Geometry: final body of the model. Coordinates: model frame, mm. A direction names the side the tool comes from. Give positions to 0.01 mm unless a question says otherwise; leave off trailing zeros. Write each loop counter-clockwise with the first axis right and the second up, starting at its lowest first coordinate (ties: lowest second). Pieces come first, ordered by that corner, then holes.
```python
from build123d import *
from build123d.topology import SkipClean

# Parameters (mm, degrees)
BOSS_EXTRUDE1_DEPTH  = 19.05
CUT_EXTRUDE1_DEPTH   = 12.7
MIRROR2_COPY_1_DEPTH = 12.7
SKETCH6_W            = 6.35
SKETCH6_H            = 32.8168
SKETCH6_W_2          = 32.8168
SKETCH6_H_2          = 6.35
CUT_EXTRUDE2_DEPTH   = 12.7
SKETCH7_R            = 0.675
BOSS_EXTRUDE2_DEPTH  = 12.7
FILLET2_DEPTH        = 20
CUT_EXTRUDE3_DEPTH   = 12.7


with BuildPart() as part:
    # Sketch5 → Boss-Extrude1 (new body)
    with BuildSketch(Plane.XY):
        with BuildLine():
            Line((-15.875, 15.875), (-15.875, -15.875))
            Line((-15.875, -15.875), (15.875, -15.875))
            ThreePointArc((15.875, -15.875), (26.071916674, -9.061638106), (38.1, -6.669103576))
            Line((38.1, -6.669103576), (38.1, 6.669103576))
            ThreePointArc((38.1, 6.669103576), (15.875, 15.875), (6.669103576, 38.1))
            Line((6.669103576, 38.1), (-6.669103576, 38.1))
            ThreePointArc((-6.669103576, 38.1), (-9.061638106, 26.071916674), (-15.875, 15.875))
        make_face()
    extrude(amount=BOSS_EXTRUDE1_DEPTH)

    # Sketch4 → Cut-Extrude1 (cut)
    with BuildSketch(Plane.XY):
        with BuildLine():
            Line((4.190365, -12.7), (10.11729625, -12.7))
            Line((10.11729625, -12.7), (12.7, -12.7))
            Line((12.7, -12.7), (12.7, -10.11729625))
            Line((12.7, -10.11729625), (12.7, -4.190365))
            Line((12.7, -4.190365), (12.7, -2.6162))
            Line((12.7, -2.6162), (11.760835, -2.6162))
            Line((11.760835, -2.6162), (11.429365, -2.6162))
            Line((11.429365, -2.6162), (9.8552, -2.6162))
            Line((9.8552, -2.6162), (9.8552, -4.190365))
            Line((9.8552, -4.190365), (9.8552, -6.348478019))
            ThreePointArc((9.8552, -6.348478019), (9.587703162, -6.748815328), (9.115473107, -6.65488293))
            Line((9.115473107, -6.65488293), (5.748911934, -3.288321756))
            ThreePointArc((5.748911934, -3.288321756), (5.404234588, -2.772475655), (5.2832, -2.16399369))
            Line((5.2832, -2.16399369), (5.2832, 0.635))
            Line((5.2832, 0.635), (1.863267895, 0.635))
            ThreePointArc((1.863267895, 0.635), (1.391939699, -1.391939699), (-0.635, -1.863267895))
            Line((-0.635, -1.863267895), (-0.635, -5.2832))
            Line((-0.635, -5.2832), (2.16399369, -5.2832))
            ThreePointArc((2.16399369, -5.2832), (2.772475655, -5.404234588), (3.288321756, -5.748911934))
            Line((3.288321756, -5.748911934), (6.65488293, -9.115473107))
            ThreePointArc((6.65488293, -9.115473107), (6.748815328, -9.587703162), (6.348478019, -9.8552))
            Line((6.348478019, -9.8552), (4.190365, -9.8552))
            Line((4.190365, -9.8552), (2.6162, -9.8552))
            Line((2.6162, -9.8552), (2.6162, -11.429365))
            Line((2.6162, -11.429365), (2.6162, -11.760835))
            Line((2.6162, -11.760835), (2.6162, -12.7))
            Line((2.6162, -12.7), (4.190365, -12.7))
        make_face()
    cut_extrude1 = extrude(amount=CUT_EXTRUDE1_DEPTH, mode=Mode.SUBTRACT)

    # Mirror1: Cut-Extrude1 across plane
    add(cut_extrude1.mirror(Plane.ZX), mode=Mode.SUBTRACT)

    # Mirror2: Cut-Extrude1 across plane
    add(cut_extrude1.mirror(Plane(origin=(0, 0, 0), x_dir=(0, 0, 1), z_dir=(1, 0, 0))), mode=Mode.SUBTRACT)

    # Mirror2 copy 1 sketch → Mirror2 copy 1 (cut)
    with BuildSketch(Plane(origin=(0, 0, 0), x_dir=(-1, 0, 0), z_dir=(0, 0, 1))):
        with BuildLine():
            Line((4.190365, -12.7), (10.11729625, -12.7))
            Line((10.11729625, -12.7), (12.7, -12.7))
            Line((12.7, -12.7), (12.7, -10.11729625))
            Line((12.7, -10.11729625), (12.7, -4.190365))
            Line((12.7, -4.190365), (12.7, -2.6162))
            Line((12.7, -2.6162), (11.760835, -2.6162))
            Line((11.760835, -2.6162), (11.429365, -2.6162))
            Line((11.429365, -2.6162), (9.8552, -2.6162))
            Line((9.8552, -2.6162), (9.8552, -4.190365))
            Line((9.8552, -4.190365), (9.8552, -6.348478019))
            ThreePointArc((9.8552, -6.348478019), (9.587703162, -6.748815328), (9.115473107, -6.65488293))
            Line((9.115473107, -6.65488293), (5.748911934, -3.288321756))
            ThreePointArc((5.748911934, -3.288321756), (5.404234588, -2.772475655), (5.2832, -2.16399369))
            Line((5.2832, -2.16399369), (5.2832, 0.635))
            Line((5.2832, 0.635), (1.863267895, 0.635))
            ThreePointArc((1.863267895, 0.635), (1.391939699, -1.391939699), (-0.635, -1.863267895))
            Line((-0.635, -1.863267895), (-0.635, -5.2832))
            Line((-0.635, -5.2832), (2.16399369, -5.2832))
            ThreePointArc((2.16399369, -5.2832), (2.772475655, -5.404234588), (3.288321756, -5.748911934))
            Line((3.288321756, -5.748911934), (6.65488293, -9.115473107))
            ThreePointArc((6.65488293, -9.115473107), (6.748815328, -9.587703162), (6.348478019, -9.8552))
            Line((6.348478019, -9.8552), (4.190365, -9.8552))
            Line((4.190365, -9.8552), (2.6162, -9.8552))
            Line((2.6162, -9.8552), (2.6162, -11.429365))
            Line((2.6162, -11.429365), (2.6162, -11.760835))
            Line((2.6162, -11.760835), (2.6162, -12.7))
            Line((2.6162, -12.7), (4.190365, -12.7))
        make_face()
    extrude(amount=MIRROR2_COPY_1_DEPTH, mode=Mode.SUBTRACT)

    # Sketch6 → Cut-Extrude2 (cut)
    with BuildSketch(Plane(origin=(0, 0, 0), x_dir=(-1, 0, 0), z_dir=(0, 0, -1))):
        with Locations((0, 21.6916)):
            Rectangle(SKETCH6_W, SKETCH6_H)
        with Locations((-21.6916, 0)):
            Rectangle(SKETCH6_W_2, SKETCH6_H_2)
    extrude(amount=-CUT_EXTRUDE2_DEPTH, mode=Mode.SUBTRACT)

    # Sketch7 → Boss-Extrude2 (add)
    with SkipClean():  # the faces are left unmerged after this step: merging them gives an invalid solid
        with BuildSketch(Plane(origin=(0, 0, 0), x_dir=(-1, 0, 0), z_dir=(0, 0, -1))):
            with Locations((-37.425, 3.175)):
                Circle(SKETCH7_R)
            with Locations((-13.375, 3.175)):
                Circle(SKETCH7_R)
            with Locations((-13.375, -3.175)):
                Circle(SKETCH7_R)
            with Locations((-37.425, -3.175)):
                Circle(SKETCH7_R)
            with Locations((-3.175, 13.375)):
                Circle(SKETCH7_R)
            with Locations((3.175, 13.375)):
                Circle(SKETCH7_R)
            with Locations((-3.175, 37.425)):
                Circle(SKETCH7_R)
            with Locations((3.175, 37.425)):
                Circle(SKETCH7_R)
            with Locations((-25.4, 3.175)):
                Circle(SKETCH7_R)
            with Locations((-25.4, -3.175)):
                Circle(SKETCH7_R)
            with Locations((-3.175, 25.4)):
                Circle(SKETCH7_R)
            with Locations((3.175, 25.4)):
                Circle(SKETCH7_R)
        extrude(amount=-BOSS_EXTRUDE2_DEPTH)

    # Fillet2: read off the stored shape, not the designer's step
    # Fillet2 outline → Fillet2 (cut)
    with SkipClean():  # the faces are left unmerged after this step: merging them gives an invalid solid
        with BuildSketch(Plane.XY):
            with BuildLine():
                Line((-15.875, -15.875), (-9.525, -15.875))
                ThreePointArc((-9.525, -15.875), (-14.015128061, -14.015128061), (-15.875, -9.525))
                Line((-15.875, -9.525), (-15.875, -15.875))
            make_face()
            with BuildLine():
                ThreePointArc((32.817272188, -7.11622946), (35.449191883, -6.781084528), (38.1, -6.669103576))
                Line((38.1, -6.669103576), (38.1, -0.85656253))
                ThreePointArc((38.1, -0.85656253), (36.602817656, -4.952006438), (32.817272188, -7.11622946))
            make_face()
            with BuildLine():
                ThreePointArc((-6.669103576, 38.1), (-6.781084528, 35.449191883), (-7.11622946, 32.817272188))
                ThreePointArc((-7.11622946, 32.817272188), (-4.952006438, 36.602817656), (-0.85656253, 38.1))
                Line((-0.85656253, 38.1), (-6.669103576, 38.1))
            make_face()
            with BuildLine():
                Line((38.1, 0.85656253), (38.1, 6.669103576))
                ThreePointArc((38.1, 6.669103576), (35.449191883, 6.781084528), (32.817272188, 7.11622946))
                ThreePointArc((32.817272188, 7.11622946), (36.602817656, 4.952006438), (38.1, 0.85656253))
            make_face()
            with BuildLine():
                ThreePointArc((0.85656253, 38.1), (4.952006438, 36.602817656), (7.11622946, 32.817272188))
                ThreePointArc((7.11622946, 32.817272188), (6.781084528, 35.449191883), (6.669103576, 38.1))
                Line((6.669103576, 38.1), (0.85656253, 38.1))
            make_face()
        extrude(amount=FILLET2_DEPTH, mode=Mode.SUBTRACT)

    # Sketch8 → Cut-Extrude3 (cut)
    with SkipClean():  # the faces are left unmerged after this step: merging them gives an invalid solid
        with BuildSketch(Plane(origin=(0, 0, 0), x_dir=(-1, 0, 0), z_dir=(0, 0, -1))):
            Polygon((-11.115734746, 10.664446616), (-11.115734746, -10.290263943), (-3.470097109, -3.989692187), (-3.470097109, 3.514359567), (3.609196999, 3.514359567), (10.051354637, 10.664446616), align=None)
        extrude(amount=-CUT_EXTRUDE3_DEPTH, mode=Mode.SUBTRACT)


solid = part.part
```
Item 1: Reachability of faces 4 (the face through (-15.875, 3, 9)), 5 (the face through (-2.5, 13.4, 6.3)) from +Z, -Z, +X, -X, +Y, -Y: full face, straight path, thin tool, end or side. Return the list, or none.
Found:
face 4: +Z, -Z, -X, +Y, -Y
face 5: -Z
Item 2: Pull-direction query (Y, two-part tool) for faces 1 (the face through (1, -7, 0)), 2 (the face through (35.861, 5.696, 9.392)), 3 (the face through (12.7, -8, 6)); classes: +Y half, -Y half, draft (parallel to the pull), parting line (faces both ways), or undercut.
Found:
face 1: draft
face 2: +Y half
face 3: undercut
Item 3: Section D-D, the plane z = 6.75. State how many separate pieces and enclosed holes the cut face has, plus the area to 3 significant figures.
Found:
separate pieces: 3
enclosed holes: 0
area: 996 mm2
Item 4: Section B-B, the plane z = 17.25. Return the cut outline in (x, y) (3 decimals).
Found:
outline: (-15.875, -9.525) arc R6.35 ccw to (-9.525, -15.875) - (15.875, -15.875) arc R31.431 cw to (32.817, -7.116) arc R6.35 ccw to (38.1, -0.857) - (38.1, 0.857) arc R6.35 ccw to (32.817, 7.116) arc R31.431 cw to (7.116, 32.817) arc R6.35 ccw to (0.857, 38.1) - (-0.857, 38.1) arc R6.35 ccw to (-7.116, 32.817) arc R31.431 cw to (-15.875, 15.875) - close
Item 5: Line query: L1, parallel to Y at x = -6.5, z = 2.75 (3 decimals); L2, parallel to Y at x = -9, z = 5 (3 decimals); L3, parallel to X at y = -5, z = 9 (3 decimals). Output: solid intervals per line, ascending.
Found:
L1: y = -15.875 to -12.7, -9.828 to -8.961, -4.039 to 4.039, 12.7 to 34.661
L2: y = -15.875 to -12.7, -6.539 to 6.539, 12.7 to 26.222
L3: x = -15.875 to -12.7, -9.855 to -7.461, 12.7 to 36.562
Item 6: Pin query (flat end, axial travel): pin 1 Ø3 at (x, z) = (30, 8) entering from +Y; pin 2 Ø2.5 at (x, z) = (-12, 4.5) entering from -Y; pin 3 Ø3 at (y, z) = (6, 6.5) entering from +X. Return the tip coordinate at first contact, or that it passes through.
Found:
pin 1: stops at y = 8.17
pin 2: stops at y = -15.76
pin 3: stops at x = 36.95
Item 7: Section C-C, the plane x = 20.5. Return the cut outline in (y, z) (3 decimals).
Found:
outline: (-12.059, 0) - (-3.175, 0) - (-3.175, 12.7) - (3.175, 12.7) - (3.175, 0) - (12.059, 0) - (12.059, 19.05) - (-12.059, 19.05) - close
